Verification items for the finished model (mm, model axes). A direction names the side the tool comes from. Give positions to 0.01 mm unless a question says otherwise; leave off trailing zeros. Loops run counter-clockwise (first coordinate to the right, second up) from the corner with the lowest first, then second, coordinate; pieces in that order, holes last. Notation, with made-up numbers: (-14.75, 35.25) - (31.25, 35.25) arc R27 cw to (31.25, 69.25) - close; hole circle Ø3 at (82.25, 83). An arc over 180 degrees is marked (long way). Answer in a Markdown table with one row per item.
```python
from build123d import *

# Parameters (mm, degrees)
BOSS_EXTRUDE1_DEPTH = 38.1
SHELL1_T            = -6.35
SKETCH3_R           = 3.4925
CUT_EXTRUDE1_DEPTH  = 6.35
SKETCH4_R           = 3.4925
CUT_EXTRUDE2_DEPTH  = 59.436
SKETCH6_W           = 25.4
SKETCH6_H           = 6.35
BOSS_EXTRUDE2_DEPTH = 26.940768


with BuildPart() as part:
    # Sketch1 → Boss-Extrude1 (new body)
    with BuildSketch(Plane.XY):
        Polygon((0, 0), (176.013019973, 176.013019973), (176.013019973, 137.913019973), (38.1, 0), align=None)
    extrude(amount=BOSS_EXTRUDE1_DEPTH)

    # Shell1
    shell1_openings = [part.faces().sort_by_distance(p)[0] for p in [
        (88.006509986, 88.006509986, 19.05),
    ]]
    offset(amount=SHELL1_T, openings=shell1_openings, kind=Kind.INTERSECTION)

    # Sketch3 → Cut-Extrude1 (cut)
    with BuildSketch(Plane.XZ):
        with Locations((19.05, 19.05)):
            Circle(SKETCH3_R)
    extrude(amount=-CUT_EXTRUDE1_DEPTH, mode=Mode.SUBTRACT)

    # Sketch4 → Cut-Extrude2 (cut)
    with BuildSketch(Plane(origin=(176.013019973, 0, 0), x_dir=(0, 0, -1), z_dir=(1, 0, 0))):
        with Locations((-19.05, 156.963019973)):
            Circle(SKETCH4_R)
    extrude(amount=-CUT_EXTRUDE2_DEPTH, mode=Mode.SUBTRACT)

    # Sketch6 → Boss-Extrude2 (add)
    with BuildSketch(Plane(origin=(0, 0, 0), x_dir=(0, 0, 1), z_dir=(-0.707106781, 0.707106781, 0))):
        with Locations((19.05, 124.333)):
            Rectangle(SKETCH6_W, SKETCH6_H)
        with Locations((19.05, 175.133)):
            Rectangle(SKETCH6_W, SKETCH6_H)
        with Locations((19.05, 73.533)):
            Rectangle(SKETCH6_W, SKETCH6_H)
    extrude(amount=-BOSS_EXTRUDE2_DEPTH)


solid = part.part
```
Q1. Go/stop test with flat-tipped pins: P1, Ø6, axis at y = 53, z = 30, coming from the +X side; P2, Ø8, axis at x = 75, z = 17.5, coming from the +Y side; P3, Ø12.5, axis at y = 148, z = 24.5, coming from the -X side; P4, Ø6.5, axis at x = 19.05, z = 19.05, coming from the -Y side. Record where each tip stops, or that it passes through.
Completed:
| item | result |
|---|---|
| P1 | x = 94.1 |
| P2 | y = 49.88 |
| P3 | x = 169.66 |
| P4 | through |
Q2. Sectioned sample at D-D (x = 113). Record the cut outline in (y, z).
Completed:
| item | result |
|---|---|
| outline | (74.9, 0) - (113, 0) - (113, 6.35) - (83.88, 6.35) - (83.88, 31.75) - (113, 31.75) - (113, 38.1) - (74.9, 38.1) - close |
Q3. Thickness scan on line 1 (Z direction, x = 19, y = 2); line 2 (X direction, y = 150, z = 17); line 3 (Y direction, x = 171, z = 19). Record the ranges inside material, lowest first.
Completed:
| item | result |
|---|---|
| line 1 | 0 to 15.56, 22.54 to 38.1 |
| line 2 | 169.66 to 176.01 |
| line 3 | 132.9 to 153.47, 160.46 to 171 |
Q4. Draft check along Y on faces 1 (the face through (24, 0, 19)), 2 (the face through (89, 89, 15)), 3 (the face through (176.013, 153, 19)), 4 (the face through (113, 99, 6.35)). Enter one of: +Y half, -Y half, draft (parallel to the pull), parting line (faces both ways), or undercut.
Completed:
| item | result |
|---|---|
| face 1 | -Y half |
| face 2 | +Y half |
| face 3 | draft |
| face 4 | undercut |
Q5. Tool access check on faces 5 (the face through (128.771, 114.415, 18.872)), 6 (the face through (97.34, 82.984, 18.872)), 7 (the face through (120.66, 91.54, 18.87)). Record the directions out of +Z, -Z, +X, -X, +Y, -Y that give a thin tool (end or side, any length) a straight path to the whole face; none if there is none.
Completed:
| item | result |
|---|---|
| face 5 | -X |
| face 6 | +Y |
| face 7 | none |
Q6. Sectioned sample at A-A (z = 19.05). Record the cut outline in (x, y).
Completed:
| item | result |
|---|---|
| outline | (0, 0) - (15.56, 0) - (15.56, 6.35) - (6.35, 6.35) - close; (22.54, 0) - (38.1, 0) - (176.01, 137.91) - (176.01, 153.47) - (169.66, 153.47) - (169.66, 140.54) - (140.64, 111.52) - (126.08, 126.08) - (121.59, 121.59) - (136.15, 107.03) - (104.72, 75.6) - (90.16, 90.16) - (85.67, 85.67) - (100.23, 71.11) - (68.8, 39.68) - (54.24, 54.24) - (49.75, 49.75) - (64.31, 35.19) - (35.47, 6.35) - (22.54, 6.35) - close; (169.66, 160.46) - (176.01, 160.46) - (176.01, 176.01) - (169.66, 169.66) - close |
Q7. Sectioned sample at B-B (x = 19.05). Record the cut outline in (y, z).
Completed:
| item | result |
|---|---|
| outline | (0, 0) - (19.05, 0) - (19.05, 6.35) - (6.35, 6.35) - (6.35, 15.56) - (0, 15.56) - close; (0, 22.54) - (6.35, 22.54) - (6.35, 31.75) - (19.05, 31.75) - (19.05, 38.1) - (0, 38.1) - close |
Q8. Sectioned sample at C-C (y = 31.5). Record the cut outline in (x, z).
Completed:
| item | result |
|---|---|
| outline | (31.5, 0) - (69.6, 0) - (69.6, 38.1) - (31.5, 38.1) - (31.5, 31.75) - (60.62, 31.75) - (60.62, 6.35) - (31.5, 6.35) - close |
